Autodesk Inventor part; units mm, degrees
ref_plane "Arbeitsebene1" through (0, 0, 0) normal (0, 1, 0) x (-1, 0, 0)
ref_plane "Arbeitsebene2" through (0, 0, 12) normal (0, 0, 1) x (1, 0, 0)
ref_plane "YZ Plane" through (0, 0, 0) normal (1, 0, 0) x (0, 1, 0)
sketch "Skizze1" plane through (0, 0, 0) normal (0, 1, 0) x (-1, 0, 0)
  line L0 (0, 19.5) -> (-30, 19.5)
  line L1 (-30, 19.5) -> (-30, -19.5)
  line L2 (-30, -19.5) -> (0, -19.5)
  line L3 (0, -19.5) -> (0, 19.5)
  line L4 (0, 6) -> (169.4, 6)
  line L5 (169.4, 6) -> (169.4, -6)
  line L6 (169.4, -6) -> (0, -6)
  line L7 (0, -6) -> (0, 6)
  line L8 (0, 0) -> (-64.3399, 0) construction
  line L9 (9, 0) -> (145, 0) construction
  line L10 (9, 3) -> (145, 3)
  line L11 (145, -3) -> (9, -3)
  arc A0 (9, 3) -> (9, -3) centre (9, 0) ccw
  arc A1 (145, -3) -> (145, 3) centre (145, 0) ccw
  point P0 (169.4, 0)
  point P1 (-15, -19.5)
  point P2 (77, 0)
  point P3 (6, 0)
  point P4 (148, 0)
  dimension "d0" = 39
  dimension "d1" = 30
  dimension "d2" = 184.4
  dimension "d3" = 12
  dimension "d4" = 6
  dimension "d5" = 6
  dimension "d6" = 3
  dimension "d27" = 142
extrude "Extrusion1" add sketch "Skizze1" along normal mid plane 12
extrude "Extrusion2" add sketch "Skizze1" along normal blind 3 contours L10 A1 L11 A0
extrude "Extrusion3" add sketch "Skizze1" against normal blind 3 contours L10 A1 L11 A0
sketch "Skizze2" plane through (0, 6, 0) normal (0, 1, 0) x (1, 0, 0)
  line L0 (30, 19.5) -> (0, 19.5)
  point P0 (0, 0)
  point P1 (15, 0)
  point P2 (15, 19.5)
hole "Bohrung1" at (15, 6, 0) direction (0, -1, 0) diameter 18 depth 12
ref_plane "Arbeitsebene1" through (0, 0, 0) normal (0, 1, 0) x (-1, 0, 0)
sketch "Skizze4" plane through (0, 0, 0) normal (0, 1, 0) x (-1, 0, 0)
  line L0 (169.4, 6) -> (169.4, -6)
  circle A0 centre (169.4, 0) radius 12
  point P0 (0, 0)
  dimension "d24" = 24
extrude "Extrusion4" add sketch "Skizze4" along normal mid plane 12
sketch "Skizze5" plane through (0, 0, 0) normal (0, 1, 0) x (-1, 0, 0)
  circle A0 centre (169.4, 0) radius 7.5
  arc A1 (159.0077, -6) -> (159.0077, 6) centre (169.4, 0) ccw
  point P0 (0, 0)
  dimension "d28" = 15
extrude "Extrusion5" cut sketch "Skizze5" along normal mid plane 12
fillet "Rundung1" radius 3 2 edges at (-159.0077, 0, 6) (-159.0077, 0, -6)
ref_plane "Arbeitsebene2" through (0, 0, 12) normal (0, 0, 1) x (1, 0, 0)
sketch "Skizze6" plane through (0, 0, 12) normal (0, 0, 1) x (1, 0, 0)
  line L0 (-181.4, -6) -> (-181.4, 6)
  line L1 (-159.8, -6) -> (-159.8, 6)
  line L2 (-159.8, -6) -> (-159.8, -6)
  line L3 (-159.8, 6) -> (-159.8, -6)
  line L4 (-159.8, 6) -> (-159.8, 6)
  line L5 (-159.8, 6) -> (-181.4, 6)
  point P0 (0, 0)
  point P1 (-170.6, 0)
  point P2 (-181.4, 0)
  point P3 (-170.6, 6)
hole "Bohrung2" at (-170.6, 0, 12) direction (0, 0, -1) diameter 6 end through all
sketch "Skizze7" plane through (0, -6, 19.5) normal (-1, 0, 0) x (0, 0, 1)
  line L0 (-12, 0) -> (-27, 0)
  line L1 (-25.5, 0) -> (-39, 0)
  line L2 (-39, 0) -> (0, 0)
  line L3 (0, 0) -> (-13.5, 0)
  line L4 (-12.3, 0) -> (-13.5, 0)
  line L5 (-12.3, 0) -> (-26.7, 0)
  line L6 (-25.5, 0) -> (-26.7, 0)
  line L7 (-22.5, 0) -> (-16.5, 0)
  line L8 (-16.5, 0) -> (-22.5, 0)
  line L9 (-10.5, 0) -> (-28.5, 0)
  point P0 (-19.5, 6)
  point P1 (-6, 6)
  point P2 (-33, 6)
  point P3 (-6.75, 0)
  dimension "d48" = 6
  dimension "d50" = 13.5
  dimension "d51" = 13.5
hole "Bohrung3" at (0, 0, 13.5) at (0, 0, -13.5) direction (1, 0, 0) diameter 6 end through all
properties part number "pleuel_rad_2"
Here's how the part is built. I have some questions about the finished solid (model axes, mm). A direction names the side the tool comes from. Round coordinates to 2 decimals unless told otherwise and drop trailing zeros. Order: outer loops, then holes, each group sorted by start corner. A loop starts at its lowest first (then second) coordinate and runs counter-clockwise, first axis right, second up. Notation, with made-up numbers: M 46,-2 L 76,-2 A29 cw 76,30 Z; hole C -1,53 d11. An arc over 180 degrees is marked long. Answer in a Markdown table with one row per item.
Item 1: Imagine slicing it at C-C, the plane x = -55.5. Write out the boundary of the cut face in (y, z).
A:
| item | result |
|---|---|
| outline | M -6,-6 L 6,-6 L 6,-3 L 3,-3 L 3,3 L 6,3 L 6,6 L -6,6 L -6,3 L -3,3 L -3,-3 L -6,-3 Z |
Item 2: I'm going to push flat-ended pins straight in: pin 1 (5 mm diameter, centred on x = -170.6, y = 0, fed in from -Z); pin 2 (6 mm diameter, centred on x = -51, y = -1.5, fed in from +Z); pin 3 (3 mm diameter, centred on y = 2.5, z = -8, fed in from -X); pin 4 (0.9 mm diameter, centred on x = -82, y = -4, fed in from -Z). Where does each tip first touch, or does it pass through?
A:
| item | result |
|---|---|
| pin 1 | passes through |
| pin 2 | stops at z = 6 |
| pin 3 | stops at x = -179.49 |
| pin 4 | stops at z = -6 |
Item 3: Thinking about a two-plate mould opening in Y: for faces 4 (the face through (-52, -6, -4)), 5 (the face through (-173.13, -1.61, -9.15)), 6 (the face through (-78, 0, 6)), which applies, +Y half, -Y half, draft (parallel to the pull), parting line (faces both ways), or undercut?
A:
| item | result |
|---|---|
| face 4 | -Y half |
| face 5 | undercut |
| face 6 | draft |
Item 4: Imagine slicing it at B-B, the plane y = 0. Write out the boundary of the cut face in (x, z), and give its area (3 significant figures).
A:
| item | result |
|---|---|
| outline | M -173.6,-11.24 L -173.6,-6.21 A7.5 cw -173.6,6.21 L -173.6,11.24 A12 ccw Z; M -167.6,-11.86 A12 ccw -159.8,-7.2 A3 cw -157.4,-6 L 0,-6 L 0,-10.5 L 30,-10.5 L 30,10.5 L 0,10.5 L 0,6 L -157.4,6 A3 cw -159.8,7.2 A12 ccw -167.6,11.86 L -167.6,7.28 A7.5 cw -167.6,-7.28 Z; M 0,-19.5 L 30,-19.5 L 30,-16.5 L 0,-16.5 Z; M 0,16.5 L 30,16.5 L 30,19.5 L 0,19.5 Z; hole C 15,0 d18 |
| area | 2,670 mm2 |
Item 5: Imagine slicing it at A-A, the plane x = 15. Write out the boundary of the cut face in (y, z).
A:
| item | result |
|---|---|
| outline | M -6,-19.5 L 6,-19.5 L 6,-9 L -6,-9 Z; M -6,9 L 6,9 L 6,19.5 L -6,19.5 Z; hole C 0,-13.5 d6; hole C 0,13.5 d6 |
Item 6: If I drill on L1, parallel to Z at x = 14.5, y = 0; L2, parallel to X at y = -4.75, z = -0.5; L3, parallel to Z at x = -94.5, y = -5, over which ranges is the centre line in solid material (lowest first)? Write a range as from..to.
A:
| item | result |
|---|---|
| L1 | z = -19.5..-16.5, -10.5..-8.99, 8.99..10.5, 16.5..19.5 |
| L2 | x = -181.39..-176.88, -161.92..-147.96, -6.04..6.01, 23.99..30 |
| L3 | z = -6..-3, 3..6 |
Item 7: For faces 1 (the face through (0, 0, -10)), 2 (the face through (-76, -3, 0)), 3 (the face through (15.2, -0.1, -16.5)), which set-ups out of +Z, -Z, +X, -X, +Y, -Y let a thin tool reach every point of the face, with its end or its side?
A:
| item | result |
|---|---|
| face 1 | -Z, +Y, -Y |
| face 2 | -Y |
| face 3 | +X |
